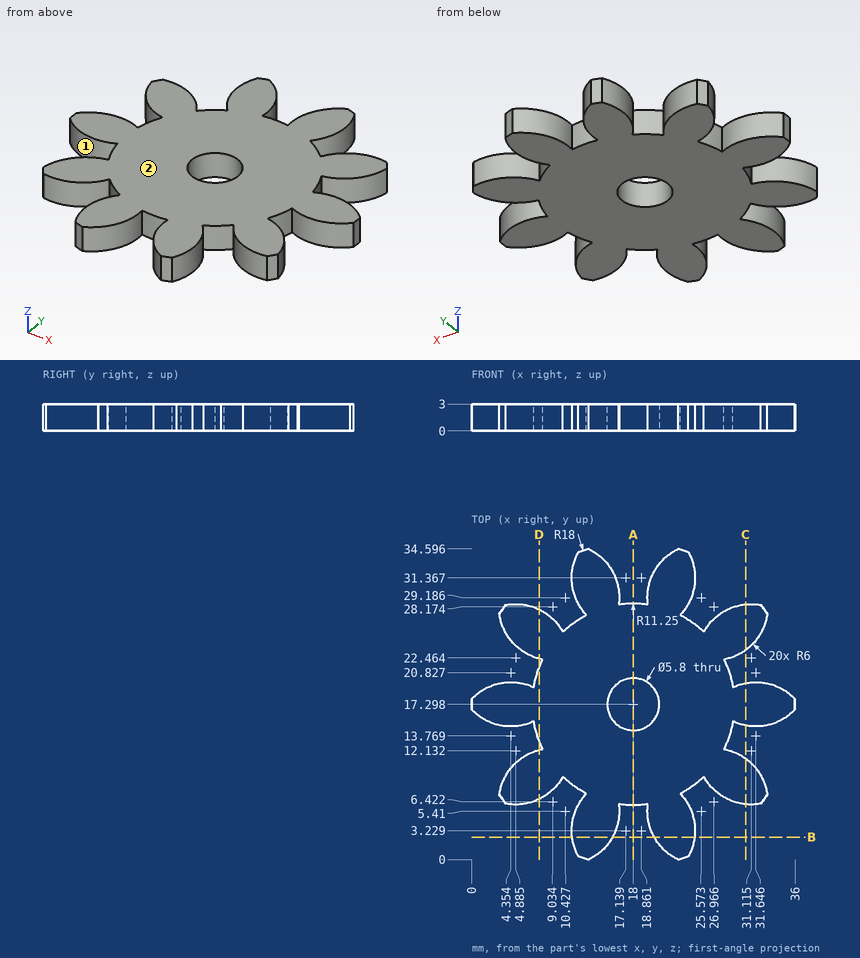
Here's the drawing with two shaded views (mm, measured from the low corner). I have some questions. Coordinates: 2 decimals unless noted, no trailing zeros. Loops run counter-clockwise (first coordinate to the right, second up) from the corner with the lowest first, then second, coordinate; pieces in that order, holes last. Notation, with made-up numbers: (-8, -17) -> (51, -17) arc R26 ccw to (51, -2) -> close; hole circle Ø9 at (16.25, -7). An arc over 180 degrees is marked (long way). Answer in a Markdown table with one row per item.
(1) Imagine slicing it at C-C (x = 30.5). List the corners of the cut face in (y, z) for me (1 decimal).
Results found:
| item | result |
|---|---|
| outline | (6.2, 0) -> (11.3, 0) -> (11.3, 3) -> (6.2, 3) -> close; (14.9, 0) -> (19.7, 0) -> (19.7, 3) -> (14.9, 3) -> close; (23.3, 0) -> (28.4, 0) -> (28.4, 3) -> (23.3, 3) -> close |
(2) If I drill on probe 1 along X at (y, z) = (28, 1.35) (1 decimal); probe 2 along Y at (x, z) = (13, 1.15) (1 decimal); probe 3 along X at (y, z) = (33, 1.75) (1 decimal), over which ranges is the centre line in solid material (lowest first)?
Results found:
| item | result |
|---|---|
| probe 1 | x = 3.5 to 7.2, 12.2 to 23.8, 28.8 to 32.5 |
| probe 2 | y = 0 to 34.6 |
| probe 3 | x = 11.4 to 15.1, 20.9 to 24.6 |
(3) Will these pins go through, and if not, where does the flat tip stop? pin 1 Ø1 at (y, z) = (12, 1.5) entering from +X; pin 2 Ø1 at (y, z) = (30.5, 0.5) entering from +X; pin 3 Ø1.5 at (y, z) = (28, 1.5) entering from -X.
Results found:
| item | result |
|---|---|
| pin 1 | stops at x = 30.16 |
| pin 2 | stops at x = 24.85 |
| pin 3 | stops at x = 3.09 |
(4) Imagine slicing it at A-A (x = 18). List the corners of the cut face in (y, z) for me.
Results found:
| item | result |
|---|---|
| outline | (6.05, 0) -> (14.4, 0) -> (14.4, 3) -> (6.05, 3) -> close; (20.2, 0) -> (28.55, 0) -> (28.55, 3) -> (20.2, 3) -> close |
(5) Thinking about a two-plate mould opening in Y: for the marked faces 1 and 2, which applies, released by +Y, released by -Y, zero draft, split by the parting line, or undercut?
Results found:
| item | result |
|---|---|
| face 1 | undercut |
| face 2 | zero draft |
(6) Imagine slicing it at B-B (y = 2.5). List the corners of the cut face in (x, z) for me.
Results found:
| item | result |
|---|---|
| outline | (11.18, 0) -> (15.67, 0) -> (15.67, 3) -> (11.18, 3) -> close; (20.33, 0) -> (24.82, 0) -> (24.82, 3) -> (20.33, 3) -> close |
(7) Imagine slicing it at D-D (x = 7.5). List the corners of the cut face in (y, z) for me (1 decimal).
Results found:
| item | result |
|---|---|
| outline | (6.7, 0) -> (12.2, 0) -> (12.2, 3) -> (6.7, 3) -> close; (13.3, 0) -> (21.3, 0) -> (21.3, 3) -> (13.3, 3) -> close; (22.4, 0) -> (27.9, 0) -> (27.9, 3) -> (22.4, 3) -> close |
